Check sheet for the modelled part. Datum: model origin and axes. Units: mm. A direction names the side the tool comes from. Give positions to 0.01 mm unless a question says otherwise; leave off trailing zeros. Order: outer loops, then holes, each group sorted by start corner. A loop starts at its lowest first (then second) coordinate and runs counter-clockwise, first axis right, second up. Notation, with made-up numbers: M 2.5,-26 L 49.5,-26 A17 cw 49.5,-1 Z; hole C -27.75,65 d3. An arc over 180 degrees is marked long. Answer in a Markdown table with one row per item. Add a question column.
from build123d import *

# Parameters (mm, degrees)
BOSS_EXTRUDE1_DEPTH = 1.524


with BuildPart() as part:
    # Sketch1 → Boss-Extrude1 (new body)
    with BuildSketch(Plane.XY):
        with BuildLine():
            Line((-3.235155639, -8.287391484), (-3.783555133, -13.357106433))
            ThreePointArc((-3.783555133, -13.357106433), (0, -13.028347252), (3.783555133, -13.357106433))
            Line((3.783555133, -13.357106433), (3.235155639, -8.287391484))
            Line((3.235155639, -8.287391484), (4.755175848, -8.122474118))
            Line((4.755175848, -8.122474118), (5.317484152, -13.35909326))
            Line((5.317484152, -13.35909326), (9.410610808, -13.358099847))
            Line((9.410610808, -13.358099847), (8.758889671, -7.983387544))
            Line((8.758889671, -7.983387544), (10.274936224, -7.800587713))
            Line((10.274936224, -7.800587713), (10.926657362, -13.174306602))
            ThreePointArc((10.926657362, -13.174306602), (15.10168665, -17.742358652), (17.820275176, -23.301787175))
            ThreePointArc((17.820275176, -23.301787175), (17.932389495, -16.299261358), (17.11310908, -9.343924052))
            ThreePointArc((17.11310908, -9.343924052), (14.904545185, -6.389006387), (12.979613066, -3.241955511))
            ThreePointArc((12.979613066, -3.241955511), (12.412109671, -2.2224752), (11.916873155, -1.165999455))
            ThreePointArc((11.916873155, -1.165999455), (11.893308886, 2.337529648), (10.570541154, 5.581841128))
            ThreePointArc((10.570541154, 5.581841128), (10.855213093, 9.786127154), (10.861185965, 14.000035485))
            ThreePointArc((10.861185965, 14.000035485), (7.971038383, 11.880829677), (6.515279188, 8.605963044))
            Line((6.515279188, 8.605963044), (7.415708302, 2.300096505))
            Line((7.415708302, 2.300096505), (5.907609567, 2.085505398))
            Line((5.907609567, 2.085505398), (4.304137007, 13.321734283))
            ThreePointArc((4.304137007, 13.321734283), (2.229613922, 15.888650106), (0.940042002, 18.926693413))
            ThreePointArc((0.940042002, 18.926693413), (1.007296175, 17.568367421), (0.751408616, 16.232667535))
            Line((0.751408616, 16.232667535), (0.753449362, 6.933674836))
            Line((0.753449362, 6.933674836), (-0.753449362, 6.933674836))
            Line((-0.753449362, 6.933674836), (-0.751408616, 16.232667535))
            ThreePointArc((-0.751408616, 16.232667535), (-1.007296175, 17.568367421), (-0.940042002, 18.926693413))
            ThreePointArc((-0.940042002, 18.926693413), (-2.229613922, 15.888650106), (-4.304137007, 13.321734283))
            Line((-4.304137007, 13.321734283), (-5.907609567, 2.085505398))
            Line((-5.907609567, 2.085505398), (-7.415708302, 2.300096505))
            Line((-7.415708302, 2.300096505), (-6.515279188, 8.605963044))
            ThreePointArc((-6.515279188, 8.605963044), (-7.971038383, 11.880829677), (-10.861185965, 14.000035485))
            ThreePointArc((-10.861185965, 14.000035485), (-10.855213093, 9.786127154), (-10.570541154, 5.581841128))
            ThreePointArc((-10.570541154, 5.581841128), (-11.893308886, 2.337529648), (-11.916873155, -1.165999455))
            ThreePointArc((-11.916873155, -1.165999455), (-12.412109671, -2.2224752), (-12.979613066, -3.241955511))
            ThreePointArc((-12.979613066, -3.241955511), (-14.904545185, -6.389006387), (-17.11310908, -9.343924052))
            ThreePointArc((-17.11310908, -9.343924052), (-17.932389495, -16.299261358), (-17.820275176, -23.301787175))
            ThreePointArc((-17.820275176, -23.301787175), (-15.10168665, -17.742358652), (-10.926657362, -13.174306602))
            Line((-10.926657362, -13.174306602), (-10.274936224, -7.800587713))
            Line((-10.274936224, -7.800587713), (-8.758889671, -7.983387544))
            Line((-8.758889671, -7.983387544), (-9.410610808, -13.358099847))
            Line((-9.410610808, -13.358099847), (-5.317484152, -13.35909326))
            Line((-5.317484152, -13.35909326), (-4.755175848, -8.122474118))
            Line((-4.755175848, -8.122474118), (-3.235155639, -8.287391484))
        make_face()
    extrude(amount=BOSS_EXTRUDE1_DEPTH)


solid = part.part
Q1. Tool access check on faces 4 (the flat face through (9.506, -7.893, 0.751)), 5 (the flat face through (-10.605, -10.525, 0.751)), 6 (the flat face through (-5.095, 7.782, 0.751)). Record the directions out of +Z, -Z, +X, -X, +Y, -Y that give a thin tool (end or side, any length) a straight path to the whole face; none if there is none.
Q2. Cross-section at C-C (y = 4.5). Record the boundary of the cut face in (x, z).
Q3. Thickness scan on probe 1 along X at (y, z) = (10.5, 0.15); probe 2 along X at (y, z) = (-12.5, 0.2); probe 3 along X at (y, z) = (-12, 1.35). Record the ranges inside material, lowest first.
Q4. Cross-section at A-A (y = 12). Record the boundary of the cut face in (x, z).
Q5. Go/stop test with flat-tipped pins: pin 1 (0.8 mm diameter, centred on x = 8, z = 0.5, fed in from -Y); pin 2 (0.8 mm diameter, centred on y = 10, z = 0.5, fed in from +X). Record where each tip stops, or that it passes through.
Q6. Cross-section at D-D (x = 8). Record the boundary of the cut face in (y, z), and give its area (3 significant figures).
Q7. Draft check along X on faces 1 (the flat face through (10.596, -10.45, 0.751)), 2 (the cylindrical face through (17.937, -16.397, 0.751)), 3 (the cylindrical face through (-12.4, -2.2, 0.8)). Enter one of: pulls with the +X half, pulls with the -X half, needs draft (parallel to the pull), parting line crosses it, or undercut.
Q8. Cross-section at B-B (y = -12). Record the boundary of the cut face in (x, z).
Values follow:
| question | item | result |
|---|---|---|
| 1 | face 4 | +Z, -Z |
| 1 | face 5 | +Z, -Z, -Y |
| 1 | face 6 | +Z, -Z, +Y |
| 2 | outline | M -11.18,0 L -7.1,0 L -7.1,1.52 L -11.18,1.52 Z; M -5.56,0 L 5.56,0 L 5.56,1.52 L -5.56,1.52 Z; M 7.1,0 L 11.18,0 L 11.18,1.52 L 7.1,1.52 Z |
| 3 | probe 1 | -10.88 to -7.1, -4.71 to -0.75, 0.75 to 4.71, 7.1 to 10.88 |
| 3 | probe 2 | -17.6 to -10.84, -9.31 to -5.23, -3.69 to 3.69, 5.23 to 9.31, 10.84 to 17.6 |
| 3 | probe 3 | -17.54 to -10.78, -9.25 to -5.17, -3.64 to 3.64, 5.17 to 9.25, 10.78 to 17.54 |
| 4 | outline | M -10.89,0 L -8.07,0 L -8.07,1.52 L -10.89,1.52 Z; M -4.49,0 L -0.75,0 L -0.75,1.52 L -4.49,1.52 Z; M 0.75,0 L 4.49,0 L 4.49,1.52 L 0.75,1.52 Z; M 8.07,0 L 10.89,0 L 10.89,1.52 L 8.07,1.52 Z |
| 5 | pin 1 | y = -13.36 |
| 5 | pin 2 | x = 10.87 |
| 6 | outline | M -13.36,0 L 11.92,0 L 11.92,1.52 L -13.36,1.52 Z |
| 6 | area | 38.5 mm² |
| 7 | face 1 | undercut |
| 7 | face 2 | pulls with the +X half |
| 7 | face 3 | pulls with the -X half |
| 8 | outline | M -17.54,0 L -10.78,0 L -10.78,1.52 L -17.54,1.52 Z; M -9.25,0 L -5.17,0 L -5.17,1.52 L -9.25,1.52 Z; M -3.64,0 L 3.64,0 L 3.64,1.52 L -3.64,1.52 Z; M 5.17,0 L 9.25,0 L 9.25,1.52 L 5.17,1.52 Z; M 10.78,0 L 17.54,0 L 17.54,1.52 L 10.78,1.52 Z |
